from build123d import *

# Parameters (mm, degrees)
SKETCH1_W           = 32
SKETCH1_H           = 69.5
SKETCH1_R           = 5
SKETCH1_R_2         = 2.25
BOSS_EXTRUDE1_DEPTH = 15
SKETCH7_W           = 40
SKETCH7_H           = 16
BOSS_EXTRUDE6_DEPTH = 15
SKETCH5_R           = 2.25
CUT_EXTRUDE2_DEPTH  = 60.052942348
CHAMFER1_SIZE       = 4


with BuildPart() as part:
    # Sketch1 → Boss-Extrude1 (new body)
    with BuildSketch(Plane(origin=(0, 0, 0), x_dir=(1, 0, 0), z_dir=(0, 1, 0))):
        with Locations((0, 18.75)):
            Rectangle(SKETCH1_W, SKETCH1_H)
        with Locations(Location((0, 0, 0), (0, 0, 270))):
            Circle(SKETCH1_R, mode=Mode.SUBTRACT)
        with Locations(Location((11.313708499, -11.313708499, 0), (0, 0, 270))):
            Circle(SKETCH1_R_2, mode=Mode.SUBTRACT)
        with Locations(Location((11.313708499, 11.313708499, 0), (0, 0, 270))):
            Circle(SKETCH1_R_2, mode=Mode.SUBTRACT)
        with Locations(Location((-11.313708499, 11.313708499, 0), (0, 0, 270))):
            Circle(SKETCH1_R_2, mode=Mode.SUBTRACT)
        with Locations(Location((-11.313708499, -11.313708499, 0), (0, 0, 270))):
            Circle(SKETCH1_R_2, mode=Mode.SUBTRACT)
    extrude(amount=BOSS_EXTRUDE1_DEPTH)

    # Sketch7 → Boss-Extrude6 (add)
    with BuildSketch(Plane(origin=(0, 0, 0), x_dir=(1, 0, 0), z_dir=(0, 1, 0))):
        with Locations((0, 45.5)):
            Rectangle(SKETCH7_W, SKETCH7_H)
    extrude(amount=BOSS_EXTRUDE6_DEPTH)

    # Sketch5 → Cut-Extrude2 (cut, through all)
    with BuildSketch(Plane(origin=(0, 0, 0), x_dir=(1, 0, 0), z_dir=(0, 1, 0))):
        with Locations(Location((0, 43.25, 0), (0, 0, 270))):
            Circle(SKETCH5_R)
        with Locations(Location((14.05, 46.25, 0), (0, 0, 270))):
            Circle(SKETCH5_R)
        with Locations(Location((-14.05, 46.25, 0), (0, 0, 270))):
            Circle(SKETCH5_R)
    extrude(amount=CUT_EXTRUDE2_DEPTH, mode=Mode.SUBTRACT)

    # Chamfer1
    chamfer1_edges = [part.edges().sort_by_distance(p)[0] for p in [
        (16, 7.5, 16),
        (-16, 7.5, 16),
        (-16, 7.5, -37.5),
        (16, 7.5, -37.5),
        (20, 7.5, -53.5),
        (-20, 7.5, -53.5),
    ]]
    chamfer(chamfer1_edges, length=CHAMFER1_SIZE - 0.0001)  # a hair under: the kernel refuses the full size


solid = part.part
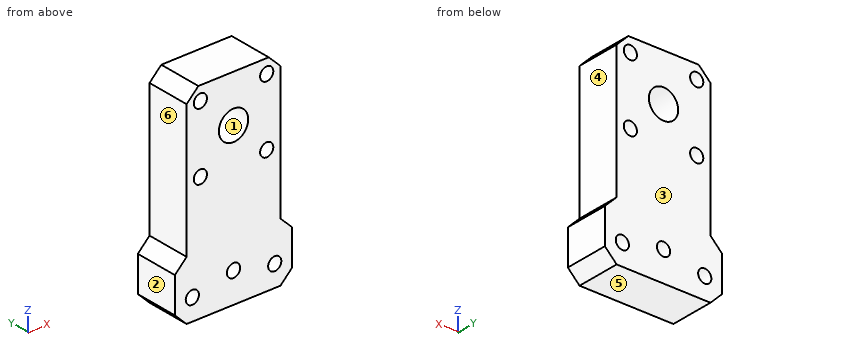
The model under review builds one solid part; all positions refer to its coordinate system, in mm. Face numbers are marked on the shaded views. A direction names the side the tool comes from. Coordinates: 2 decimals unless noted, no trailing zeros. Order: outer loops, then holes, each group sorted by start corner. A loop starts at its lowest first (then second) coordinate and runs counter-clockwise, first axis right, second up. Notation, with made-up numbers: (47, 37.25) -> (106, 37.25) arc R17 cw to (106, 51.25) -> close; hole circle Ø9 at (88, 27.5). An arc over 180 degrees is marked (long way). Answer in a Markdown table with one row per item.
(1) Insertion check: pin 1 (6 mm diameter, centred on y = 6.5, z = 0.5, fed in from +X); pin 2 (8 mm diameter, centred on y = 9, z = 8.5, fed in from -X). Each pin has a flat end and moves straight along its axis. Give the tip position at first contact, or say it passes through.
Answers:
| item | result |
|---|---|
| pin 1 | x = 16 |
| pin 2 | x = -16 |
(2) The part is to be moulded in two halves that separate along X. For the marked faces 1, 2 and 3, say which applies: +X half, -X half, draft (parallel to the pull), parting line (faces both ways), or undercut.
Answers:
| item | result |
|---|---|
| face 1 | undercut |
| face 2 | -X half |
| face 3 | draft |
(3) Consider section A-A (z = 0). Write out the cut boundary in (x, y), plus the area to 3 significant figures.
Answers:
| item | result |
|---|---|
| outline | (-16, 0) -> (-5, 0) -> (-5, 15) -> (-16, 15) -> close; (5, 0) -> (16, 0) -> (16, 15) -> (5, 15) -> close |
| area | 330 mm² |
(4) Machinability: for the marked faces 4, 5 and 6, which of the approach directions +Z, -Z, +X, -X, +Y, -Y give a long, thin tool a straight path to every point of the face, cutting with its end or side? Answer none if there is none.
Answers:
| item | result |
|---|---|
| face 4 | +Z, +X, +Y, -Y |
| face 5 | -Z, +X, -X, +Y, -Y |
| face 6 | +Z, -X, +Y, -Y |
(5) Consider section B-B (x = 0). Write out the cut boundary in (y, z).
Answers:
| item | result |
|---|---|
| outline | (0, -53.5) -> (15, -53.5) -> (15, -45.5) -> (0, -45.5) -> close; (0, -41) -> (15, -41) -> (15, -5) -> (0, -5) -> close; (0, 5) -> (15, 5) -> (15, 16) -> (0, 16) -> close |
(6) Consider section D-D (y = 3.75). State how many separate pieces and enclosed holes the cut face has, plus the area to 3 significant figures.
Answers:
| item | result |
|---|---|
| separate pieces | 1 |
| enclosed holes | 8 |
| area | 2,150 mm² |
(7) Consider section C-C (z = -47.5). Write out the cut boundary in (x, y), plus the area to 3 significant figures.
Answers:
| item | result |
|---|---|
| outline | (-20, 0) -> (-15.92, 0) -> (-15.92, 15) -> (-20, 15) -> close; (-12.18, 0) -> (12.18, 0) -> (12.18, 15) -> (-12.18, 15) -> close; (15.92, 0) -> (20, 0) -> (20, 15) -> (15.92, 15) -> close |
| area | 488 mm² |
(8) Wall thickness on line 1 along X through (y, z) = (7.75, -46); line 2 along Z through (x, y) = (13, 6); line 3 along Z through (x, y) = (2, 6.5): over which ranges is each line inside the solid? List them lowest first.
Answers:
| item | result |
|---|---|
| line 1 | -20 to -16.29, -11.81 to 11.81, 16.29 to 20 |
| line 2 | -53.5 to -48.24, -44.26 to -12.8, -9.82 to 9.82, 12.8 to 15 |
| line 3 | -53.5 to -44.28, -42.22 to -4.58, 4.58 to 16 |
